```python
from build123d import *

# Parameters (mm, degrees)
BOSS_EXTRUDE1_DEPTH = 30
SKETCH4_R           = 1.5
SKETCH4_R_2         = 2.5
CUT_EXTRUDE1_DEPTH  = 49.076771644
CUT_EXTRUDE3_DEPTH  = 31.802137849


with BuildPart() as part:
    # Sketch2 → Boss-Extrude1 (new body)
    with BuildSketch(Plane.XY):
        Polygon((-18.901068924, 20), (-18.901068924, 14), (12.901068924, 14), (12.901068924, -14), (-18.901068924, -14), (-18.901068924, -20), (18.901068924, -20), (18.901068924, 20), align=None)
    extrude(amount=BOSS_EXTRUDE1_DEPTH)

    # Sketch4 → Cut-Extrude1 (cut, through all)
    with BuildSketch(Plane.ZY.offset(-12.901068924)):
        with Locations((15, 8)):
            Circle(SKETCH4_R)
        with Locations((15, 0)):
            Circle(SKETCH4_R_2)
        with Locations((15, -8)):
            Circle(SKETCH4_R)
        with Locations((5.5, 0)):
            Circle(SKETCH4_R)
        with Locations((24.5, 0)):
            Circle(SKETCH4_R)
    extrude(amount=-CUT_EXTRUDE1_DEPTH, mode=Mode.SUBTRACT)

    # Sketch7 → Cut-Extrude3 (cut)
    with BuildSketch(Plane.ZY.offset(18.901068924)):
        with BuildLine():
            Line((0, -14), (30, -14))
            add(Edge.make_bspline(
                [(0, -14), (5, -14.51661298), (15, -15.549838941), (25, -14.51661298), (30, -14)],
                knots=[0, 0, 0, 0, 0.5, 1, 1, 1, 1], degree=3))
        make_face()
        with BuildLine():
            Line((0, 14), (30, 14))
            add(Edge.make_bspline(
                [(0, 14), (5, 14.51661298), (15, 15.549838941), (25, 14.51661298), (30, 14)],
                knots=[0, 0, 0, 0, 0.5, 1, 1, 1, 1], degree=3))
        make_face()
    extrude(amount=-CUT_EXTRUDE3_DEPTH, mode=Mode.SUBTRACT)


solid = part.part
```
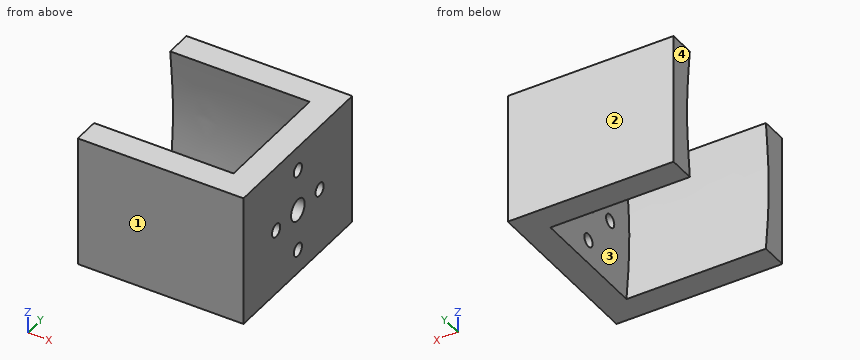
Verification items for the finished model (mm, model axes). Face numbers are marked on the shaded views. Round coordinates to 2 decimals unless told otherwise and drop trailing zeros. Write each loop counter-clockwise with the first axis right and the second up, starting at its lowest first coordinate (ties: lowest second). Pieces come first, ordered by that corner, then holes.
1. Section check A-A on z = 15. State how many separate pieces and enclosed holes the cut face has, plus the area to 3 significant figures.
2. Section check B-B on y = -5. Enter the section's corners in (x, z), plus the area to 3 significant figures.
3. Scan lines: L1, parallel to Y at x = 14, z = 15; L2, parallel to Y at x = 5, z = 14; L3, parallel to X at y = 10.5, z = 28. Record each from-to range of solid material in increasing order.
4. Draft check along Y on the marked faces 1, 2, 3 and 4. Enter one of: +Y half, -Y half, draft (parallel to the pull), parting line (faces both ways), or undercut.
5. Gauge pin test, flat end, axial feed: P1, Ø1, axis at y = 0, z = 11, coming from the -X side. Record the tip position at first contact, or that the pin passes through.
Answer:
1. separate pieces: 4
1. enclosed holes: 0
1. area: 490 mm2
2. outline: (12.9, 0) - (18.9, 0) - (18.9, 30) - (12.9, 30) - close
2. area: 180 mm2
3. L1: y = -20 to -9.5, -6.5 to -2.5, 2.5 to 6.5, 9.5 to 20
3. L2: y = -20 to -15.03, 15.03 to 20
3. L3: x = 12.9 to 18.9
4. face 1: -Y half
4. face 2: +Y half
4. face 3: undercut
4. face 4: draft
5. P1: stops at x = 12.9
